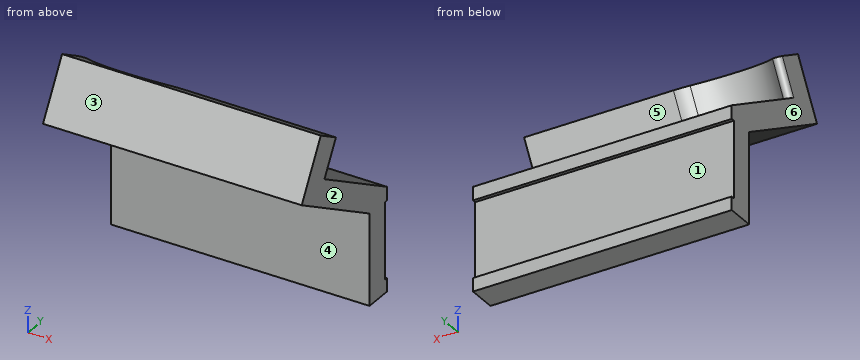
```python
from build123d import *

# Parameters (mm, degrees)
BOSS_EXTRUDE1_DEPTH = 80
CUT_EXTRUDE1_DEPTH  = 50
CUT_EXTRUDE2_DEPTH  = 101.49080803735235
BOSS_EXTRUDE2_REACH = 102.491
CUT_EXTRUDE10_DEPTH = 50
SKETCH6_R           = 13.750000000000007
CUT_EXTRUDE3_DEPTH  = 102.06821275824429
CUT_EXTRUDE4_DEPTH  = 101.49080803735237
SKETCH8_R           = 6.000000000000003
CUT_EXTRUDE5_DEPTH  = 73.15845701593427
CUT_EXTRUDE6_DEPTH  = 73.15845701593429
CUT_EXTRUDE7_DEPTH  = 69.27999960632745
FILLET5_R           = 1
FILLET6_R           = 5
CUT_EXTRUDE8_DEPTH  = 67.6997627150144
BOSS_EXTRUDE4_DEPTH = 22
BOSS_EXTRUDE5_DEPTH = 55
CUT_EXTRUDE9_DEPTH  = 0.75
BOSS_EXTRUDE6_DEPTH = 55


with BuildPart() as part:
    # Sketch1 → Boss-Extrude1 (new body)
    with BuildSketch(Plane(origin=(0, 0, 0), x_dir=(1, 0, 0), z_dir=(0, 1, 0))):
        Polygon((-1e-17, 25.95), (55, 25.95), (55.00000000000001, 0), (0, 0), align=None)
    extrude(amount=BOSS_EXTRUDE1_DEPTH)

    # Sketch4 → Cut-Extrude1 (cut)
    with BuildSketch(Plane(origin=(55.00000000000001, 0, -1.471e-14), x_dir=(0, 0, -1), z_dir=(1, 0, 0))):
        Polygon((-77.30254037844365, 60.0000000000004), (-27.30254037844327, 146.60254037844405), (59.300000000000374, 96.60254037844365), (9.299999999999985, 9.999999999999995), align=None)
    extrude(amount=-CUT_EXTRUDE1_DEPTH, mode=Mode.SUBTRACT)

    # Sketch5 → Cut-Extrude2 (cut, through all)
    with BuildSketch(Plane(origin=(55.00000000000001, 0, -1.471e-14), x_dir=(0, 0, -1), z_dir=(1, 0, 0))):
        Polygon((-11.160254037844386, 10.265727792645105), (-6.160254037844387, 18.92598183048949), (2.4999999999999942, 13.925981830489496), (-2.499999999999998, 5.265727792645102), align=None)
    extrude(amount=-CUT_EXTRUDE2_DEPTH, mode=Mode.SUBTRACT)

    # Sketch12 → Boss-Extrude2 (add, up to next)
    with BuildSketch(Plane(origin=(55.00000000000001, 0, -1.471e-14), x_dir=(0, 0, -1), z_dir=(1, 0, 0)), mode=Mode.PRIVATE) as boss_extrude2_sk1:
        Polygon((2.4999999999999942, 13.925981830489496), (9.299999999999985, 9.999999999999995), (9.800000000000008, 10.866025403784473), (2.9999999999999933, 14.792007234273935), align=None)
    boss_extrude2_tool1 = extrude(boss_extrude2_sk1.sketch, amount=-BOSS_EXTRUDE2_REACH, mode=Mode.PRIVATE) - part.part
    add(boss_extrude2_tool1.solids().sort_by_distance((55, 12.396004, -6.15))[0])

    # Sketch21 → Cut-Extrude10 (cut)
    with BuildSketch(Plane(origin=(55.00000000000001, 0, -1.471e-14), x_dir=(-2.7e-16, 0, -1), z_dir=(1, 0, -2.7e-16))):
        Polygon((3.0000000000000075, 14.792007234273937), (2.2500000000000036, 13.49296912859728), (9.050000000000018, 9.566987298107822), (9.800000000000008, 10.866025403784464), align=None)
    extrude(amount=-CUT_EXTRUDE10_DEPTH, mode=Mode.SUBTRACT)

    # Sketch6 → Cut-Extrude3 (cut, through all)
    with BuildSketch(Plane(origin=(0, -1.5270181275976227, -2.6448729810777505), x_dir=(1, 0, 0), z_dir=(0, 0.5000000000000042, 0.8660254037844363))):
        with Locations((12.000000000000004, 22.810254037844377)):
            Circle(SKETCH6_R)
    extrude(amount=CUT_EXTRUDE3_DEPTH, mode=Mode.SUBTRACT)

    # Sketch7 → Cut-Extrude4 (cut, through all)
    with BuildSketch(Plane(origin=(55.00000000000001, 0, -1.471e-14), x_dir=(0, 0, -1), z_dir=(1, 0, 0))):
        Polygon((-1.613e-14, 9.595854811567275), (3.8935696044755734, 16.339715189324856), (10.693569604475588, 12.413733358835394), (66.80169358562932, 109.59585481156728), (25.408423261372093, 109.59585481156728), (-1e-17, 109.59585481156728), align=None)
    extrude(amount=-CUT_EXTRUDE4_DEPTH, mode=Mode.SUBTRACT)

    # Sketch8 → Cut-Extrude5 (cut, through all)
    with BuildSketch(Plane(origin=(0, 0, 0), x_dir=(1, 0, 0), z_dir=(0, 1, 0))):
        with Locations((25.749999999999996, 27.449999999999996)):
            Circle(SKETCH8_R)
    extrude(amount=CUT_EXTRUDE5_DEPTH, mode=Mode.SUBTRACT)

    # Sketch9 → Cut-Extrude6 (cut, through all)
    with BuildSketch(Plane(origin=(55.00000000000001, 0, -1.471e-14), x_dir=(0, 0, -1), z_dir=(1, 0, 0))):
        Polygon((21.449999999999978, 31.044417311961634), (25.94999999999998, 31.044417311961634), (25.94999999999998, 38.8386459460215), align=None)
    extrude(amount=-CUT_EXTRUDE6_DEPTH, mode=Mode.SUBTRACT)

    # Sketch10 → Cut-Extrude7 (cut, through all)
    with BuildSketch(Plane(origin=(0, 0, 0), x_dir=(1, 0, 0), z_dir=(0, 1, 0))):
        Polygon((55.00000000000001, 21.449999999999992), (0, 21.449999999999996), (0, 25.94999999999999), (55.00000000000001, 25.949999999999992), align=None)
    extrude(amount=CUT_EXTRUDE7_DEPTH, mode=Mode.SUBTRACT)

    # Fillet5
    fillet5_edges = [part.edges().sort_by_distance(p)[0] for p in [
        (0, 14.37672427408014, -7.293569604475611),
    ]]
    fillet(fillet5_edges, radius=FILLET5_R)

    # Fillet6
    fillet6_edges = [part.edges().sort_by_distance(p)[0] for p in [
        (21.437293044088527, 11.52997821335257, -5.650000000000027),
    ]]
    fillet(fillet6_edges, radius=FILLET6_R)

    # Sketch16 → Cut-Extrude8 (cut, through all)
    with BuildSketch(Plane(origin=(55.00000000000001, 0, -1.471e-14), x_dir=(0, 0, -1), z_dir=(1, 0, 0))):
        Polygon((21.44999999999998, 20.54441731196163), (11.346633369868394, 3.04487298107776), (-1.613e-14, 9.595854811567275), (1.8e-15, 0), (21.44999999999998, 0), align=None)
    extrude(amount=-CUT_EXTRUDE8_DEPTH, mode=Mode.SUBTRACT)

    # Sketch17 → Boss-Extrude4 (add)
    with BuildSketch(Plane(origin=(1.35e-15, 0, -21.449999999999996), x_dir=(-1, 0, 0), z_dir=(0, 0, -1))):
        Polygon((-55.00000000000001, 31.044417311961634), (1.35e-15, 31.044417311961634), (7.2e-16, 25.044417311961638), (-55.00000000000001, 25.044417311961638), align=None)
    extrude(amount=BOSS_EXTRUDE4_DEPTH)

    # Sketch18 → Boss-Extrude5 (add)
    with BuildSketch(Plane(origin=(55.00000000000001, 0, -1.471e-14), x_dir=(-2.4e-16, 0, -1), z_dir=(1, 0, -2.4e-16))):
        Polygon((16.39831668493419, 11.794645146519695), (27.51217782649105, 31.044417311961634), (21.449999999999978, 31.044417311961634), (11.8516833150658, 14.419645146519745), align=None)
    extrude(amount=-BOSS_EXTRUDE5_DEPTH)

    # Sketch19 → Cut-Extrude9 (cut)
    with BuildSketch(Plane(origin=(0, 31.044417311961634, 0), x_dir=(1, 0, 0), z_dir=(0, 1, 0))):
        Polygon((1e-15, 40.599999999999994), (55.00000000000001, 40.6), (55.00000000000001, 24.29999999999999), (2e-15, 24.29999999999999), align=None)
    extrude(amount=-CUT_EXTRUDE9_DEPTH, mode=Mode.SUBTRACT)

    # Sketch20 → Boss-Extrude6 (add)
    with BuildSketch(Plane(origin=(55.00000000000001, 0, -1.471e-14), x_dir=(-2.4e-16, 0, -1), z_dir=(1, 0, -2.4e-16))):
        Polygon((-1.613e-14, 9.595854811567275), (-0.7500000000000167, 8.296816705890615), (10.59663336986839, 1.7458348754011042), (11.346633369868393, 3.04487298107776), align=None)
    extrude(amount=-BOSS_EXTRUDE6_DEPTH)


solid = part.part
```
Geometry check sheet. Reference: the model listing, model coordinates, mm. Face numbers are marked on the shaded views. A direction names the side the tool comes from. Give positions to 0.01 mm unless a question says otherwise; leave off trailing zeros. Order: outer loops, then holes, each group sorted by start corner. A loop starts at its lowest first (then second) coordinate and runs counter-clockwise, first axis right, second up. Notation, with made-up numbers: (49.5, -32.75) -> (69.5, -32.75) arc R23 cw to (69.5, 5.25) -> close; hole circle Ø1 at (-14.5, -25). An arc over 180 degrees is marked (long way). Write each question's results on one line, items separated by ' | '. Start each with the question number.
(1) Sectioned sample at B-B (z = -27.5). Enter the section's corners in (x, y).
(2) Sectioned sample at A-A (x = 38.5). Enter the section's corners in (y, z).
(3) Gauge pin test, flat ends, axial feed: P1, Ø4, axis at x = 33.5, z = -20.5, coming from the -Y side; P2, Ø12, axis at x = 14, y = 18, coming from the -Z side; P3, Ø1, axis at x = 40, y = 11, coming from the +Z side; P4, Ø13, axis at x = 19, z = -29.5, coming from the +Y side. Record the tip position at first contact, or that the pin passes through.
(4) Access from +Z, -Z, +X, -X, +Y, -Y to the whole of each face (thin tool, end or side, straight path). Record for the marked faces 4, 5 and 6.
(5) Scan lines: line 1 (Y direction, x = 32, z = -30); line 2 (Z direction, x = 17, y = 10.25); line 3 (Z direction, x = 28, y = 12.5). Record each from-to range of solid material in increasing order.
(6) Sectioned sample at D-D (x = 13.5). Enter the section's corners in (y, z).
(7) Sectioned sample at C-C (y = 21.5). Enter the section's corners in (x, z).
(8) Mould release check, pull along Z, two halves, no side actions. Record for the marked faces 1, 2 and 3: pulls with the +Z half, pulls with the -Z half, needs draft (parallel to the pull), parting line crosses it, or undercut.
Answer below:
1) outline: (0, 25.04) -> (55, 25.04) -> (55, 30.29) -> (0, 30.29) -> close
2) outline: (1.75, -10.6) -> (25.04, -24.05) -> (25.04, -43.45) -> (31.04, -43.45) -> (31.04, -40.6) -> (30.29, -40.6) -> (30.29, -24.3) -> (31.04, -24.3) -> (31.04, -21.45) -> (9.57, -9.05) -> (13.49, -2.25) -> (8.3, 0.75) -> close
3) P1: y = 15.43 | P2: z = -23.45 | P3: z = -0.52 | P4: y = 31.04
4) face 4: -Z, +X, -X, -Y | face 5: +X, +Y | face 6: +Z, -Z, -X, +Y, -Y
5) line 1: 25.04 to 30.29 | line 2: -15.51 to -9.44, -2.25 to -0.38 | line 3: -16.81 to -10.74, -3.97 to -1.68
6) outline: (1.75, -10.6) -> (25.04, -24.05) -> (25.04, -43.45) -> (31.04, -43.45) -> (31.04, -40.6) -> (30.29, -40.6) -> (30.29, -24.3) -> (31.04, -24.3) -> (31.04, -21.45) -> (6.39, -7.22) -> (10.32, -0.42) -> (8.3, 0.75) -> close
7) outline: (0, -22) -> (55, -22) -> (55, -15.94) -> (0, -15.94) -> close
8) face 1: undercut | face 2: needs draft | face 3: pulls with the +Z half
